Part model, mm, in its own coordinate system. A direction names the side the tool comes from. Give positions to 0.01 mm unless a question says otherwise; leave off trailing zeros. Order: outer loops, then holes, each group sorted by start corner. A loop starts at its lowest first (then second) coordinate and runs counter-clockwise, first axis right, second up.
1. Probe line 1 (Z direction, x = -15.5, y = 9.75); line 2 (X direction, y = 9.25, z = 0); line 3 (Z direction, x = 15, y = 9.5). List the from-to ranges inside material, lowest first.
2. Slice it at A-A on z = 0. List the corners of the cut face in (x, y), and give its area (3 significant figures).
3. Mould opens along X. For faces 1 (the cylindrical face through (-23.567, 7.056, -14.586)), 2 (the flat face through (-28.5, 6, 0)), 3 (the flat face through (-27, 1, -18.5)) say: +X half, -X half, draft (parallel to the pull), parting line (faces both ways), or undercut.
4. Slice it at C-C on y = 1. Give the number of separate pieces and of enclosed holes in the cut face, and give its area (3 significant figures).
5. Which spindle directions (+Z, -Z, +X, -X, +Y, -Y) get a long thin tool onto all of the face, cutting with end or side? Do faces 4 (the cylindrical face through (-27.07, 5.58, -27)), 5 (the flat face through (27, 1, 12.5)), 6 (the cylindrical face through (15.4, 1.5, -22)), 7 (the flat face through (-16, 3, 27)). Say none if no direction does.
6. Slice it at B-B on x = 0. List the corners of the cut face in (y, z).
7. Drop flat-ended pins along their axis: pin 1 Ø4.5 at (x, z) = (-25, -15.5) entering from +Y; pin 2 Ø2 at (x, z) = (25, 15.5) entering from -Y; pin 3 Ø1.5 at (y, z) = (1, -26.5) entering from -X. Give the stop position or say it passes through.
from build123d import *

# Parameters (mm, degrees)
SKETCH_1_W                           = 57
SKETCH_1_H                           = 57
EXTRUDE_1_DEPTH                      = 11
FILLET_1_R                           = 5
SKETCH_2_R                           = 27
CUT_EXTRUDE_1_DEPTH                  = 3
SKETCH_3_R                           = 25.05
CUT_EXTRUDE_2_DEPTH                  = 6
SKETCH_4_R                           = 23.5
CUT_EXTRUDE_3_DEPTH                  = 2
CHAMFER_1_SIZE                       = 1
SKETCH_5_R                           = 2.5
SKETCH_5_R_2                         = 1.7
CUT_EXTRUDE_4_DEPTH                  = 42.779181419
EXTRUDE_2_DEPTH                      = 1
CHAMFER_2_SIZE                       = 0.2
CUT_EXTRUDE_5_DEPTH                  = 3
PATTERN_CIRCULAR_1_COUNT             = 4
CHAMFER_2_OF_PATTERN_CIRCULAR_1_SIZE = 0.2


with BuildPart() as part:
    # 草图1 → 凸台-拉伸1 (new body)
    with BuildSketch(Plane(origin=(0, 0, 0), x_dir=(1, 0, 0), z_dir=(0, 1, 0))):
        Rectangle(SKETCH_1_W, SKETCH_1_H)
    extrude(amount=EXTRUDE_1_DEPTH)

    # 圆角1
    fillet_1_edges = [part.edges().sort_by_distance(p)[0] for p in [
        (28.5, 5.5, 28.5),
        (-28.5, 5.5, 28.5),
        (-28.5, 5.5, -28.5),
        (28.5, 5.5, -28.5),
    ]]
    fillet(fillet_1_edges, radius=FILLET_1_R)

    # 草图2 → 切除-拉伸1 (cut)
    with BuildSketch(Plane(origin=(0, 11, 0), x_dir=(1, 0, 0), z_dir=(0, 1, 0))):
        with Locations(Location((0, 0, 0), (0, 0, 270))):
            Circle(SKETCH_2_R)
    extrude(amount=-CUT_EXTRUDE_1_DEPTH, mode=Mode.SUBTRACT)

    # 草图3 → 切除-拉伸2 (cut)
    with BuildSketch(Plane(origin=(0, 8, 0), x_dir=(1, 0, 0), z_dir=(0, 1, 0))):
        with Locations(Location((0, 0, 0), (0, 0, 270))):
            Circle(SKETCH_3_R)
    extrude(amount=-CUT_EXTRUDE_2_DEPTH, mode=Mode.SUBTRACT)

    # 草图4 → 切除-拉伸3 (cut)
    with BuildSketch(Plane(origin=(0, 2, 0), x_dir=(1, 0, 0), z_dir=(0, 1, 0))):
        with Locations(Location((0, 0, 0), (0, 0, 270))):
            Circle(SKETCH_4_R)
    extrude(amount=-CUT_EXTRUDE_3_DEPTH, mode=Mode.SUBTRACT)

    # 倒角1
    chamfer_1_edges = [part.edges().sort_by_distance(p)[0] for p in [
        (0, 8, -25.05),
    ]]
    chamfer(chamfer_1_edges, length=CHAMFER_1_SIZE)

    # 草图5 → 切除-拉伸4 (cut, through all)
    with BuildSketch(Plane(origin=(0, 11, 0), x_dir=(1, 0, 0), z_dir=(0, 1, 0))):
        with Locations(Location((-23.5, 23.5, 0), (0, 0, 270))):
            Circle(SKETCH_5_R)
        with Locations(Location((-25, 15.5, 0), (0, 0, 270))):
            Circle(SKETCH_5_R_2)
    cut_extrude_4 = extrude(amount=-CUT_EXTRUDE_4_DEPTH, mode=Mode.SUBTRACT)

    # 草图6 → 凸台-拉伸2 (add)
    with BuildSketch(Plane(origin=(0, 11, 0), x_dir=(1, 0, 0), z_dir=(0, 1, 0))):
        Polygon((-28.5, 11), (-28.5, -11), (-27.5, -10), (-27.5, 10), align=None)
    extrude_2 = extrude(amount=EXTRUDE_2_DEPTH)

    # 倒角2
    chamfer_2_edges = [part.edges().sort_by_distance(p)[0] for p in [
        (-27.5, 12, 0),
    ]]
    chamfer(chamfer_2_edges, length=CHAMFER_2_SIZE)

    # 草图7 → 切除-拉伸5 (cut)
    with BuildSketch(Plane.XZ):
        with BuildLine():
            Line((-25, -18.5), (-30.818208661, -18.5))
            ThreePointArc((-30.818208661, -18.5), (-33.818208661, -15.5), (-30.818208661, -12.5))
            Line((-30.818208661, -12.5), (-25, -12.5))
            ThreePointArc((-25, -12.5), (-22, -15.5), (-25, -18.5))
        make_face()
    cut_extrude_5 = extrude(amount=-CUT_EXTRUDE_5_DEPTH, mode=Mode.SUBTRACT)

    # 阵列(圆周)1: 切除-拉伸4, 凸台-拉伸2, 切除-拉伸5 ×4 about axis
    pattern_circular_1_axis = Axis((0, 0, 0), (0, 1, 0))
    add([cut_extrude_4.rotate(pattern_circular_1_axis, i * 360 / PATTERN_CIRCULAR_1_COUNT) for i in range(1, PATTERN_CIRCULAR_1_COUNT)], mode=Mode.SUBTRACT)
    add([extrude_2.rotate(pattern_circular_1_axis, i * 360 / PATTERN_CIRCULAR_1_COUNT) for i in range(1, PATTERN_CIRCULAR_1_COUNT)])
    add([cut_extrude_5.rotate(pattern_circular_1_axis, i * 360 / PATTERN_CIRCULAR_1_COUNT) for i in range(1, PATTERN_CIRCULAR_1_COUNT)], mode=Mode.SUBTRACT)

    # 倒角2 of 阵列(圆周)1
    chamfer_2_of_pattern_circular_1_edges = [part.edges().sort_by_distance(p)[0] for p in [
        (0, 12, 27.5),
        (27.5, 12, 0),
        (0, 12, -27.5),
    ]]
    chamfer(chamfer_2_of_pattern_circular_1_edges, length=CHAMFER_2_OF_PATTERN_CIRCULAR_1_SIZE)


solid = part.part
Data:
1. line 1: z = -28.5 to -22.11, 22.11 to 23.3, 26.7 to 28.5
1. line 2: x = -28.5 to -27, 27 to 28.5
1. line 3: z = -28.5 to -26.62, -23.38 to -22.45, 22.45 to 28.5
2. outline: (-28.5, 0) - (-23.5, 0) - (-23.5, 2) - (-25.05, 2) - (-25.05, 7) - (-26.05, 8) - (-27, 8) - (-27, 11) - (-27.5, 11) - (-27.5, 11.8) - (-27.7, 12) - (-28.5, 12) - close; (23.5, 0) - (28.5, 0) - (28.5, 12) - (27.7, 12) - (27.5, 11.8) - (27.5, 11) - (27, 11) - (27, 8) - (26.05, 8) - (25.05, 7) - (25.05, 2) - (23.5, 2) - close
2. area: 71.4 mm2
3. face 1: undercut
3. face 2: -X half
3. face 3: draft
4. separate pieces: 1
4. enclosed holes: 5
4. area: 1,270 mm2
5. face 4: -Z, -X, +Y, -Y
5. face 5: +X, -Y
5. face 6: -Z, -Y
5. face 7: +Z, -Y
6. outline: (0, -28.5) - (12, -28.5) - (12, -27.7) - (11.8, -27.5) - (11, -27.5) - (11, -27) - (8, -27) - (8, -26.05) - (7, -25.05) - (2, -25.05) - (2, -23.5) - (0, -23.5) - close; (0, 23.5) - (2, 23.5) - (2, 25.05) - (7, 25.05) - (8, 26.05) - (8, 27) - (11, 27) - (11, 27.5) - (11.8, 27.5) - (12, 27.7) - (12, 28.5) - (0, 28.5) - close
7. pin 1: stops at y = 11
7. pin 2: passes through
7. pin 3: stops at x = -27.97
